Build history of the part. All positions in model axes, mm. Face numbers are marked on the shaded views. Give positions to 0.01 mm unless a question says otherwise; leave off trailing zeros. Order: outer loops, then holes, each group sorted by start corner. A loop starts at its lowest first (then second) coordinate and runs counter-clockwise, first axis right, second up. Notation, with made-up numbers: (-9.75, 3) - (47.25, 3) arc R30 cw to (47.25, 26) - close; hole circle Ø8 at (-11.75, 20). An arc over 180 degrees is marked (long way). Write each question's results on one line, items separated by ' | '. Start each with the question number.
1) Drop flat-ended pins along their axis: pin 1 Ø10.5 at (x, z) = (0, 0) entering from +Y; pin 2 Ø2 at (x, y) = (-23.5, 1.5) entering from +Z; pin 3 Ø2 at (y, z) = (4.5, 22) entering from -X; pin 4 Ø1 at (y, z) = (1.5, 25.5) entering from +X. Give the stop position or say it passes through.
2) Cut at B-B on z = 0. List the corners of the cut face in (x, y), plus the area to 3 significant figures.
3) Cut at A-A on x = 0. List the corners of the cut face in (y, z), plus the area to 3 significant figures.
4) Cut at C-C on x = 22. List the corners of the cut face in (y, z), plus the area to 3 significant figures.
5) Two-plate mould, pull along Z, no slides. Class the marked faces 1, 2, 3 and 4: +Z half, -Z half, draft (parallel to the pull), parting line (faces both ways), or undercut.
6) Drill centre lines: line 1 along X through (y, z) = (1, 21); line 2 along Z through (x, y) = (21.5, 5); line 3 along X through (y, z) = (4.25, -19). Where is each one in solid material? Low to high. Write a range as from..to.
7) Cut at D-D on y = 1. List the corners of the cut face in (x, z) (3 decimals), plus the area to 3 significant figures.
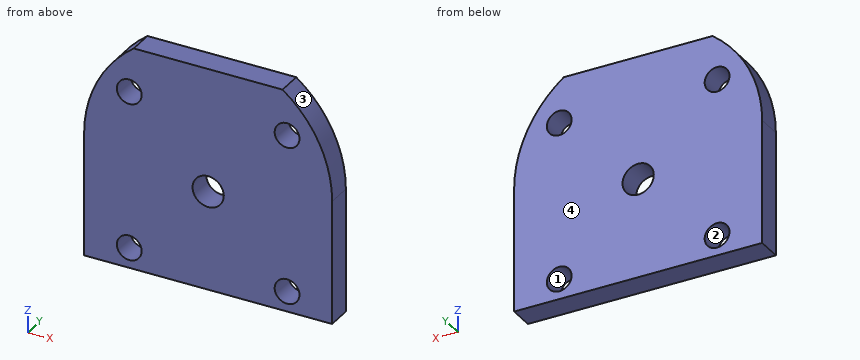
from build123d import *

# Parameters (mm, degrees)
SKETCH1_R           = 3.175
SKETCH1_R_2         = 4
BOSS_EXTRUDE1_DEPTH = 6.35


with BuildPart() as part:
    # Sketch1 → Boss-Extrude1 (new body)
    with BuildSketch(Plane(origin=(0, 0, 0), x_dir=(1, 0, 0), z_dir=(0, 1, 0))):
        with BuildLine():
            Line((-31.75, 25.4), (-31.75, 0))
            Line((-31.75, 0), (-31.75, -6.35))
            ThreePointArc((-31.75, -6.35), (-28.398063314, -20.549031657), (-19.05, -31.75))
            Line((-19.05, -31.75), (19.05, -31.75))
            ThreePointArc((19.05, -31.75), (28.398063314, -20.549031657), (31.75, -6.35))
            Line((31.75, -6.35), (31.75, 0))
            Line((31.75, 0), (31.75, 25.4))
            Line((31.75, 25.4), (-31.75, 25.4))
        make_face()
        with Locations(Location((-20.205576272, -20.205576272, 0), (0, 0, 270))):
            Circle(SKETCH1_R, mode=Mode.SUBTRACT)
        with Locations(Location((20.205576272, -20.205576272, 0), (0, 0, 270))):
            Circle(SKETCH1_R, mode=Mode.SUBTRACT)
        with Locations(Location((0, 0, 0), (0, 0, 270))):
            Circle(SKETCH1_R_2, mode=Mode.SUBTRACT)
        with Locations(Location((-20.205576272, 20.205576272, 0), (0, 0, 270))):
            Circle(SKETCH1_R, mode=Mode.SUBTRACT)
        with Locations(Location((20.205576272, 20.205576272, 0), (0, 0, 270))):
            Circle(SKETCH1_R, mode=Mode.SUBTRACT)
    extrude(amount=BOSS_EXTRUDE1_DEPTH)


solid = part.part
Results:
1) pin 1: y = 6.35 | pin 2: z = 28.75 | pin 3: x = -28.17 | pin 4: x = 25.7
2) outline: (-31.75, 0) - (-4, 0) - (-4, 6.35) - (-31.75, 6.35) - close; (4, 0) - (31.75, 0) - (31.75, 6.35) - (4, 6.35) - close | area: 352 mm^2
3) outline: (0, -25.4) - (6.35, -25.4) - (6.35, -4) - (0, -4) - close; (0, 4) - (6.35, 4) - (6.35, 31.75) - (0, 31.75) - close | area: 312 mm^2
4) outline: (0, -25.4) - (6.35, -25.4) - (6.35, -22.82) - (0, -22.82) - close; (0, -17.59) - (6.35, -17.59) - (6.35, 17.59) - (0, 17.59) - close; (0, 22.82) - (6.35, 22.82) - (6.35, 29.24) - (0, 29.24) - close | area: 280 mm^2
5) face 1: undercut | face 2: undercut | face 3: +Z half | face 4: draft
6) line 1: -28.17..-23.28, -17.13..17.13, 23.28..28.17 | line 2: -25.4..-23.1, -17.31..17.31, 23.1..29.71 | line 3: -31.75..-23.14, -17.27..17.27, 23.14..31.75
7) outline: (-31.75, -25.4) - (31.75, -25.4) - (31.75, 6.35) arc R31.75 ccw to (19.05, 31.75) - (-19.05, 31.75) arc R31.75 ccw to (-31.75, 6.35) - close; hole circle Ø6.35 at (-20.206, -20.206); hole circle Ø6.35 at (-20.206, 20.206); hole circle Ø8 at (0, 0); hole circle Ø6.35 at (20.206, -20.206); hole circle Ø6.35 at (20.206, 20.206) | area: 3,260 mm^2
